```python
from build123d import *

# Parameters (mm, degrees)
SKETCH5_R           = 20
BOSS_EXTRUDE3_DEPTH = 40
SKETCH6_R           = 7.5
CUT_EXTRUDE3_DEPTH  = 10
BOSS_EXTRUDE4_DEPTH = 2
SKETCH8_R           = 5
CUT_EXTRUDE6_DEPTH  = 25
SKETCH9_R           = 12.5
CUT_EXTRUDE7_DEPTH  = 5
SKETCH10_R          = 5
BOSS_EXTRUDE5_DEPTH = 5


with BuildPart() as part:
    # Sketch5 → Boss-Extrude3 (new body)
    with BuildSketch(Plane.XY):
        Circle(SKETCH5_R)
    extrude(amount=BOSS_EXTRUDE3_DEPTH)

    # Sketch6 → Cut-Extrude3 (cut)
    with BuildSketch(Plane.XY.offset(40)):
        Circle(SKETCH6_R)
    extrude(amount=-CUT_EXTRUDE3_DEPTH, mode=Mode.SUBTRACT)

    # Sketch7 → Boss-Extrude4 (add)
    with BuildSketch(Plane.XY.offset(40)):
        with BuildLine():
            ThreePointArc((-2, 7.228416147), (0, 7.5), (2, 7.228416147))
            Line((2, 7.228416147), (2, 14.866068747))
            ThreePointArc((2, 14.866068747), (0, 15), (-2, 14.866068747))
            Line((-2, 14.866068747), (-2, 7.228416147))
        make_face()
        with BuildLine():
            Line((11.87439319, 9.165085181), (5.259992013, 5.346258881))
            ThreePointArc((5.259992013, 5.346258881), (6.495190528, 3.75), (7.259992013, 1.882157266))
            Line((7.259992013, 1.882157266), (13.87439319, 5.700983566))
            ThreePointArc((13.87439319, 5.700983566), (12.990381057, 7.5), (11.87439319, 9.165085181))
        make_face()
        with BuildLine():
            Line((13.87439319, -5.700983566), (7.259992013, -1.882157266))
            ThreePointArc((7.259992013, -1.882157266), (6.495190528, -3.75), (5.259992013, -5.346258881))
            Line((5.259992013, -5.346258881), (11.87439319, -9.165085181))
            ThreePointArc((11.87439319, -9.165085181), (12.990381057, -7.5), (13.87439319, -5.700983566))
        make_face()
        with BuildLine():
            Line((2, -14.866068747), (2, -7.228416147))
            ThreePointArc((2, -7.228416147), (0, -7.5), (-2, -7.228416147))
            Line((-2, -7.228416147), (-2, -14.866068747))
            ThreePointArc((-2, -14.866068747), (0, -15), (2, -14.866068747))
        make_face()
        with BuildLine():
            ThreePointArc((-5.259992013, -5.346258881), (-6.495190528, -3.75), (-7.259992013, -1.882157266))
            Line((-7.259992013, -1.882157266), (-13.87439319, -5.700983566))
            ThreePointArc((-13.87439319, -5.700983566), (-12.990381057, -7.5), (-11.87439319, -9.165085181))
            Line((-11.87439319, -9.165085181), (-5.259992013, -5.346258881))
        make_face()
        with BuildLine():
            ThreePointArc((-7.259992013, 1.882157266), (-6.495190528, 3.75), (-5.259992013, 5.346258881))
            Line((-5.259992013, 5.346258881), (-11.87439319, 9.165085181))
            ThreePointArc((-11.87439319, 9.165085181), (-12.990381057, 7.5), (-13.87439319, 5.700983566))
            Line((-13.87439319, 5.700983566), (-7.259992013, 1.882157266))
        make_face()
    extrude(amount=BOSS_EXTRUDE4_DEPTH)

    # Sketch8 → Cut-Extrude6 (cut)
    with BuildSketch(Plane(origin=(0, 0, 0), x_dir=(-1, 0, 0), z_dir=(0, 0, -1))):
        Circle(SKETCH8_R)
    extrude(amount=-CUT_EXTRUDE6_DEPTH, mode=Mode.SUBTRACT)

    # Sketch9 → Cut-Extrude7 (cut)
    with BuildSketch(Plane(origin=(0, 0, 0), x_dir=(-1, 0, 0), z_dir=(0, 0, -1))):
        Circle(SKETCH9_R)
    extrude(amount=-CUT_EXTRUDE7_DEPTH, mode=Mode.SUBTRACT)

    # Sketch10 → Boss-Extrude5 (add)
    with BuildSketch(Plane.XY.offset(30)):
        Circle(SKETCH10_R)
    extrude(amount=BOSS_EXTRUDE5_DEPTH)


solid = part.part
```
Input: part model. Units: mm. Frame: model coordinates. A direction names the side the tool comes from. Give positions to 0.01 mm unless a question says otherwise; leave off trailing zeros. Loops run counter-clockwise (first coordinate to the right, second up) from the corner with the lowest first, then second, coordinate; pieces in that order, holes last.
1) Mould query, pull axis X, two halves, no side actions, for faces 1 (the flat face through (-10.613, 3.818, 40.986)), 2 (the cylindrical face through (-11.923, 3.755, 2.465)), 3 (the flat face through (10, -5, 42)). Classes: released by +X, released by -X, zero draft, split by the parting line, or undercut.
A:
face 1: released by -X
face 2: undercut
face 3: zero draft
2) Contact query for flat-ended pins moving along their axis: pin 1 (1 mm diameter, centred on y = -9.5, z = 41, fed in from +X); pin 2 (5 mm diameter, centred on x = 5, z = 9, fed in from -Y); pin 3 (10 mm diameter, centred on y = 7, z = 31.5, fed in from +X); pin 4 (5 mm diameter, centred on x = -8.5, y = 2, fed in from +Z). Output: stop coordinate, or through.
A:
pin 1: stops at x = 12
pin 2: stops at y = -19.84
pin 3: stops at x = 19.9
pin 4: stops at z = 42
3) Line query: L1, parallel to Y at x = 0, z = 33.5; L2, parallel to Y at x = 0, z = 37.25; L3, parallel to Z at x = 1, y = -10.5. Output: solid intervals per line, ascending.
A:
L1: y = -20 to -7.5, -5 to 5, 7.5 to 20
L2: y = -20 to -7.5, 7.5 to 20
L3: z = 5 to 42
4) Section query B-B on x = 0. Return the cut outline in (y, z), and give its area (4 significant figures).
A:
outline: (-20, 0) - (-12.5, 0) - (-12.5, 5) - (-5, 5) - (-5, 25) - (5, 25) - (5, 5) - (12.5, 5) - (12.5, 0) - (20, 0) - (20, 40) - (15, 40) - (15, 42) - (7.5, 42) - (7.5, 30) - (5, 30) - (5, 35) - (-5, 35) - (-5, 30) - (-7.5, 30) - (-7.5, 42) - (-15, 42) - (-15, 40) - (-20, 40) - close
area: 1,205 mm2
5) Section query A-A on z = 32.5. Return the cut outline in (x, y), and give its area (3 significant figures).
A:
outline: circle Ø40 at (0, 0); circle Ø10 at (0, 0); hole circle Ø15 at (0, 0)
area: 1,160 mm2
6) Section query C-C on y = 0. Return the cut outline in (x, z).
A:
outline: (-20, 0) - (-12.5, 0) - (-12.5, 5) - (-5, 5) - (-5, 25) - (5, 25) - (5, 5) - (12.5, 5) - (12.5, 0) - (20, 0) - (20, 40) - (7.5, 40) - (7.5, 30) - (5, 30) - (5, 35) - (-5, 35) - (-5, 30) - (-7.5, 30) - (-7.5, 40) - (-20, 40) - close
7) Section query D-D on z = 20. Return the cut outline in (x, y), and give its area (3 significant figures).
A:
outline: circle Ø40 at (0, 0); hole circle Ø10 at (0, 0)
area: 1,180 mm2
8) Reachability of faces 4 (the flat face through (8.61, 7.28, 40.99)), 5 (the flat face through (2, 11, 41)), 6 (the flat face through (0, 0, 25)), 7 (the flat face through (8.52, -7.23, 40.99)) from +Z, -Z, +X, -X, +Y, -Y: full face, straight path, thin tool, end or side. Return the list, or none.
A:
face 4: +Z, +Y
face 5: +Z, +Y, -Y
face 6: -Z
face 7: +Z, -Y
